The listing builds one solid part. Answer for the finished solid, in the listing's coordinates (mm). A direction names the side the tool comes from. Coordinates: 2 decimals unless noted, no trailing zeros. Write each loop counter-clockwise with the first axis right and the second up, starting at its lowest first coordinate (ties: lowest second). Pieces come first, ordered by that corner, then holes. Notation, with made-up numbers: M 78,77 L 119,77 A10 cw 119,85 Z; hole C 20.5,-10 d7. An arc over 180 degrees is marked long. Answer as CSV lines item,"result".
```python
from build123d import *

# Parameters (mm, degrees)
SKETCH1_R           = 6.3
SKETCH1_R_2         = 3.3
BOSS_EXTRUDE1_DEPTH = 6.35
SKETCH2_W           = 10
SKETCH2_H           = 30
SKETCH2_R           = 1.6
BOSS_EXTRUDE2_DEPTH = 4
FILLET1_R           = 2


with BuildPart() as part:
    # Sketch1 → Boss-Extrude1 (new body)
    with BuildSketch(Plane(origin=(0, 0, 0), x_dir=(1, 0, 0), z_dir=(0, 1, 0))):
        Circle(SKETCH1_R)
        Circle(SKETCH1_R_2, mode=Mode.SUBTRACT)
        with BuildLine():
            Line((-6.3, 39), (-6.3, 0))
            ThreePointArc((-6.3, 0), (0, 6.3), (6.3, 0))
            Line((6.3, 0), (6.3, 39))
            Line((6.3, 39), (-6.3, 39))
        make_face()
    extrude(amount=BOSS_EXTRUDE1_DEPTH)

    # Sketch2 → Boss-Extrude2 (add)
    with BuildSketch(Plane(origin=(0, 0, -39), x_dir=(-1, 0, 0), z_dir=(0, 0, -1))):
        with Locations((-1.3, 15)):
            Rectangle(SKETCH2_W, SKETCH2_H)
        with Locations((-1.3, 15)):
            Circle(SKETCH2_R, mode=Mode.SUBTRACT)
    extrude(amount=-BOSS_EXTRUDE2_DEPTH)

    # Fillet1
    fillet1_edges = [part.edges().sort_by_distance(p)[0] for p in [
        (6.3, 30, -37),
        (-3.7, 6.35, -37),
        (-3.7, 30, -37),
        (1.3, 6.35, -35),
    ]]
    fillet(fillet1_edges, radius=FILLET1_R)


solid = part.part
```
Q1. The mould has two halves that part along X. Classify faces 1 (the cylindrical face through (-2.43, 3.13, -2.23)), 2 (the cylindrical face through (-0.1, 3.1, 6.3)), 3 (the flat face through (1, 19, -35)), 4 (the cylindrical face through (5.73, 29.4, -36.97)): pulls with the +X half, pulls with the -X half, needs draft (parallel to the pull), parting line crosses it, or undercut.
Output:
face 1,"undercut"
face 2,"parting line crosses it"
face 3,"needs draft"
face 4,"pulls with the +X half"
Q2. Find section C-C (x = 1.3). Give the vertices of the cut face in (y, z), and give its area (3 significant figures).
Output:
outline,"M 0,-39 L 13.4,-39 L 13.4,-35 L 8.35,-35 A2 cw 6.35,-33 L 6.35,-3.03 L 0,-3.03 Z; M 0,3.03 L 6.35,3.03 L 6.35,6.16 L 0,6.16 Z; M 16.6,-39 L 30,-39 L 30,-35 L 16.6,-35 Z"
area,"331 mm2"
Q3. Flat-ended cylindrical pins translate along their axes: pin 1 Ø5 at (y, z) = (23, -31) entering from +X; pin 2 Ø1.5 at (x, z) = (2.5, -7) entering from +Y; pin 3 Ø3 at (y, z) = (15.5, -36) entering from -X; pin 4 Ø5 at (x, y) = (1.3, 15) entering from +Z. Find the tip coordinate at first contact, or state that the pin passes through.
Output:
pin 1,"through"
pin 2,"y = 6.35"
pin 3,"x = -3.7"
pin 4,"z = -35"
Q4. For faces 5 (the flat face through (6.3, 6, -22)), 6 (the flat face through (-3.7, 18, -37)), determine the directions among +Z, -Z, +X, -X, +Y, -Y from which every point of the face is accessible in a straight line to the end or side of a thin tool.
Output:
face 5,"+Z, -Z, +X, +Y, -Y"
face 6,"+Z, -Z, -X, +Y"
Q5. Find section D-D (y = 19). Give the vertices of the cut face in (x, z), and give its area (3 significant figures).
Output:
outline,"M -3.7,-39 L 6.3,-39 L 6.3,-35 L -3.7,-35 Z"
area,"40.0 mm2"
Q6. Find section B-B (z = 1). Give the vertices of the cut face in (x, y), and give its area (3 significant figures).
Output:
outline,"M -6.22,0 L -3.14,0 L -3.14,6.35 L -6.22,6.35 Z; M 3.14,0 L 6.22,0 L 6.22,6.35 L 3.14,6.35 Z"
area,"39.1 mm2"
Q7. Find section A-A (y = 15). Give the vertices of the cut face in (x, z).
Output:
outline,"M -3.7,-39 L -0.3,-39 L -0.3,-35 L -3.7,-35 Z; M 2.9,-39 L 6.3,-39 L 6.3,-35 L 2.9,-35 Z"
Q8. Straight lines are drawn through the part: line 1 (Z direction, x = 0, y = 3.25); line 2 (Y direction, x = -0.75, z = -8); line 3 (Z direction, x = 0, y = 16.25). For each, find the intervals that lie inside material, in ascending order.
Output:
line 1,"-39 to -3.3, 3.3 to 6.3"
line 2,"0 to 6.35"
line 3,"-39 to -35"
